```python
from build123d import *

# Parameters (mm, degrees)
SKETCH_1_W           = 35.5
SKETCH_1_H           = 24
EXTRUDE_1_DEPTH      = 12.5
SKETCH_2_W           = 33
SKETCH_2_H           = 22
CUT_EXTRUDE_1_DEPTH  = 11.5
CUT_EXTRUDE_2_DEPTH  = 2
EXTRUDE_2_DEPTH      = 6
SKETCH_7_W           = 4
SKETCH_7_H           = 2
SKETCH_7_W_2         = 5
EXTRUDE_3_DEPTH      = 5
CUT_EXTRUDE_4_DEPTH  = 2
SKETCH_11_R          = 0.5
CUT_EXTRUDE_5_DEPTH  = 35
SKETCH_12_W          = 5.5
SKETCH_12_H          = 1
CUT_EXTRUDE_6_DEPTH  = 5
SKETCH_15_W          = 5.5
SKETCH_15_H          = 3
CUT_EXTRUDE_7_DEPTH  = 5
SKETCH_16_W          = 5.1
SKETCH_16_H          = 3.5
CUT_EXTRUDE_8_DEPTH  = 5
SKETCH_18_W          = 7
SKETCH_18_H          = 1
FPC_DEPTH            = 2
SKETCH_19_W          = 8
SKETCH_19_H          = 12
USB_DEPTH            = 2
SKETCH_20_W          = 4
SKETCH_20_H          = 2
CUT_EXTRUDE_10_DEPTH = 2
SKETCH_21_W          = 4
SKETCH_21_H          = 1
CUT_EXTRUDE_11_DEPTH = 2


with BuildPart() as part:
    # 草图1 → 凸台-拉伸1 (new body)
    with BuildSketch(Plane.XY):
        Rectangle(SKETCH_1_W, SKETCH_1_H)
    extrude(amount=EXTRUDE_1_DEPTH)

    # 草图2 → 切除-拉伸1 (cut)
    with BuildSketch(Plane.XY.offset(12.5)):
        with Locations((0.25, 0)):
            Rectangle(SKETCH_2_W, SKETCH_2_H)
    extrude(amount=-CUT_EXTRUDE_1_DEPTH, mode=Mode.SUBTRACT)

    # 草图3 → 切除-拉伸2 (cut)
    with BuildSketch(Plane.ZY.offset(17.75)):
        with BuildLine():
            Line((6.5, 7.45), (6.5, 0.95))
            ThreePointArc((6.5, 0.95), (4.75, -0.8), (3, 0.95))
            Line((3, 0.95), (3, 7.45))
            ThreePointArc((3, 7.45), (4.75, 9.2), (6.5, 7.45))
        make_face()
    extrude(amount=-CUT_EXTRUDE_2_DEPTH, mode=Mode.SUBTRACT)

    # 草图6 → 凸台-拉伸2 (add)
    with BuildSketch(Plane.XY.offset(1)):
        Polygon((-16.25, 10), (15.75, 10), (15.75, -10), (-16.25, -10), (-16.25, -11), (16.75, -11), (16.75, 11), (-16.25, 11), align=None)
    extrude(amount=EXTRUDE_2_DEPTH)

    # 草图7 → 凸台-拉伸3 (add)
    with BuildSketch(Plane.XY.offset(1)):
        with Locations((11.25, -9)):
            Rectangle(SKETCH_7_W, SKETCH_7_H)
        with Locations((13.25, 9)):
            Rectangle(SKETCH_7_W_2, SKETCH_7_H)
    extrude(amount=EXTRUDE_3_DEPTH)

    # 草图10 → 切除-拉伸4 (cut)
    with BuildSketch(Plane.ZY.offset(-15.75)):
        with BuildLine():
            Line((2, -8), (2, 3))
            ThreePointArc((2, 3), (4, 5), (6, 3))
            Line((6, 3), (6, -8))
            ThreePointArc((6, -8), (4, -10), (2, -8))
        make_face()
    extrude(amount=-CUT_EXTRUDE_4_DEPTH, mode=Mode.SUBTRACT)

    # 草图11 → 切除-拉伸5 (cut)
    with BuildSketch(Plane(origin=(17.75, 0, 0), x_dir=(0, 0, -1), z_dir=(1, 0, 0))):
        with Locations((-11.25, -10)):
            Circle(SKETCH_11_R)
    extrude(amount=-CUT_EXTRUDE_5_DEPTH, mode=Mode.SUBTRACT)

    # 草图12 → 切除-拉伸6 (cut)
    with BuildSketch(Plane.XY.offset(7)):
        with Locations((-2, -10.5)):
            Rectangle(SKETCH_12_W, SKETCH_12_H)
    extrude(amount=-CUT_EXTRUDE_6_DEPTH, mode=Mode.SUBTRACT)

    # 草图15 → 切除-拉伸7 (cut)
    with BuildSketch(Plane(origin=(0, -11, 0), x_dir=(1, 0, 0), z_dir=(0, 1, 0))):
        with Locations((-2, -5.5)):
            Rectangle(SKETCH_15_W, SKETCH_15_H)
    extrude(amount=-CUT_EXTRUDE_7_DEPTH, mode=Mode.SUBTRACT)

    # 草图16 → 切除-拉伸8 (cut)
    with BuildSketch(Plane.XZ.offset(-10)):
        with Locations((-3.2, 5.25)):
            Rectangle(SKETCH_16_W, SKETCH_16_H)
    extrude(amount=-CUT_EXTRUDE_8_DEPTH, mode=Mode.SUBTRACT)

    # 草图18 → FPC排线间隙 (cut)
    with BuildSketch(Plane.XY.offset(7)):
        with Locations((4.25, -10.5)):
            Rectangle(SKETCH_18_W, SKETCH_18_H)
    extrude(amount=-FPC_DEPTH, mode=Mode.SUBTRACT)

    # 草图19 → USB支撑 (add)
    with BuildSketch(Plane.XY.offset(1)):
        with Locations((-12.25, 4)):
            Rectangle(SKETCH_19_W, SKETCH_19_H)
    extrude(amount=USB_DEPTH)

    # 草图20 → 切除-拉伸10 (cut)
    with BuildSketch(Plane(origin=(0, 12, 0), x_dir=(1, 0, 0), z_dir=(0, 1, 0))):
        with Locations((2.75, -8)):
            Rectangle(SKETCH_20_W, SKETCH_20_H)
    extrude(amount=-CUT_EXTRUDE_10_DEPTH, mode=Mode.SUBTRACT)

    # 草图21 → 切除-拉伸11 (cut)
    with BuildSketch(Plane.XY.offset(7)):
        with Locations((2.75, 10.5)):
            Rectangle(SKETCH_21_W, SKETCH_21_H)
    extrude(amount=-CUT_EXTRUDE_11_DEPTH, mode=Mode.SUBTRACT)


solid = part.part
```
Input: part model. Units: mm. Frame: model coordinates. A direction names the side the tool comes from. Give positions to 0.01 mm unless a question says otherwise; leave off trailing zeros. Order: outer loops, then holes, each group sorted by start corner. A loop starts at its lowest first (then second) coordinate and runs counter-clockwise, first axis right, second up. Notation, with made-up numbers: M 32,28.5 L 76,28.5 A37 ccw 76,64.5 Z; hole C 41.25,40.5 d11. An arc over 180 degrees is marked long. Return JSON: item names as keys, results as strings.
Item 1: Ray query, probe 1 along X at (y, z) = (-6.25, 6.75); probe 2 along Y at (x, z) = (6, 8.25); probe 3 along X at (y, z) = (-6.25, 11.5). Return the intervals inside material, ascending.
Solutions:
{"probe 1": "-17.75 to -16.25, 15.75 to 17.75", "probe 2": "-12 to -11, 11 to 12", "probe 3": "-17.75 to -16.25, 16.75 to 17.75"}
Item 2: Access query for faces 1 (the cylindrical face through (17.257, -10.488, 11.358)), 2 (the flat face through (-4.75, -11, 5)), 3 (the cylindrical face through (-17, -0.8, 4.8)). Directions: +Z, -Z, +X, -X, +Y, -Y. A direction counts if a zero-diameter tool reaches every point of the face in a straight line with its end or side. Return the directions, or none.
Solutions:
{"face 1": "+X", "face 2": "none", "face 3": "-X"}
Item 3: Cut plane B-B (y = -3.5). Return loops of the section in (x, z), then the cut area to 4 significant figures.
Solutions:
{"outline": "M -17.75,0 L 17.75,0 L 17.75,2 L 15.75,2 L 15.75,1 L -16.25,1 L -16.25,12.5 L -17.75,12.5 Z; M 15.75,6 L 17.75,6 L 17.75,12.5 L 16.75,12.5 L 16.75,7 L 15.75,7 Z", "area": "62.25 mm^2"}
Item 4: Cut plane A-A (x = -2.5). Return loops of the section in (y, z).
Solutions:
{"outline": "M -12,0 L 12,0 L 12,3.5 L 10,3.5 L 10,1 L -10,1 L -10,2 L -11,2 L -11,4 L -12,4 Z; M -12,7 L -11,7 L -11,12.5 L -12,12.5 Z; M 11,7 L 12,7 L 12,12.5 L 11,12.5 Z"}
Item 5: First-contact query: P1, Ø3, axis at x = -2.5, y = 7, coming from the -Z side; P2, Ø2, axis at x = 12, y = 2.5, coming from the +Z side; P3, Ø2, axis at x = -11.5, y = 4, coming from the +Z side. Flat tips, straight axial feed; report the tip coordinate or a pass-through.
Solutions:
{"P1": "z = 0", "P2": "z = 1", "P3": "z = 3"}
Item 6: Pull-direction query (X, two-part tool) for faces 4 (the flat face through (-2, -10.5, 2)), 5 (the flat face through (0, 12, 6)); classes: +X half, -X half, draft (parallel to the pull), parting line (faces both ways), or undercut.
Solutions:
{"face 4": "undercut", "face 5": "draft"}
Item 7: Cut plane D-D (x = 11.5). Return loops of the section in (y, z).
Solutions:
{"outline": "M -12,0 L 12,0 L 12,12.5 L 11,12.5 L 11,7 L 10,7 L 10,6 L 8,6 L 8,1 L -8,1 L -8,6 L -10,6 L -10,7 L -11,7 L -11,12.5 L -12,12.5 Z"}
Item 8: Cut plane C-C (z = 11.25). Return loops of the section in (x, y).
Solutions:
{"outline": "M -17.75,-12 L 17.75,-12 L 17.75,-10.5 L 16.75,-10.5 L 16.75,-11 L -16.25,-11 L -16.25,-10.5 L -17.25,-10.5 L -17.25,-9.5 L -16.25,-9.5 L -16.25,11 L 16.75,11 L 16.75,-9.5 L 17.75,-9.5 L 17.75,12 L -17.75,12 Z"}
